Geometry check sheet. Reference: the model listing, model coordinates, mm. Face numbers are marked on the shaded views. Coordinates: 2 decimals unless noted, no trailing zeros. Loops run counter-clockwise (first coordinate to the right, second up) from the corner with the lowest first, then second, coordinate; pieces in that order, holes last. Notation, with made-up numbers: (25.5, -4) -> (79.5, -4) arc R13 cw to (79.5, 1) -> close; hole circle Ø4 at (6.5, -25.5). An arc over 180 degrees is marked (long way). Answer as a JSON object with one key per item and string values.
from build123d import *

# Parameters (mm, degrees)
SKETCH_1_W                       = 240
SKETCH_1_H                       = 160
EXTRUDE_1_DEPTH                  = 32
SKETCH_3_R                       = 13.5
CUT_EXTRUDE_2_DEPTH              = 291.213714355
PATTERN_LINEAR_5_COUNT           = 2
PATTERN_LINEAR_5_PITCH           = 80
PATTERN_LINEAR_6_COUNT           = 2
PATTERN_LINEAR_6_PITCH           = 80
PATTERN_LINEAR_7_COUNT           = 2
PATTERN_LINEAR_7_PITCH           = 80
PATTERN_LINEAR_7_COPY_1_SKETCH_R = 13.5
PATTERN_LINEAR_7_COPY_1_DEPTH    = 291.213714355
PATTERN_LINEAR_7_COPY_2_SKETCH_R = 13.5
PATTERN_LINEAR_7_COPY_2_DEPTH    = 291.213714355


with BuildPart() as part:
    # 草图1 → 凸台-拉伸1 (new body)
    with BuildSketch(Plane(origin=(0, 0, 0), x_dir=(1, 0, 0), z_dir=(0, 1, 0))):
        with Locations((120, 80)):
            Rectangle(SKETCH_1_W, SKETCH_1_H)
    extrude(amount=EXTRUDE_1_DEPTH)

    # 草图3 → 切除-拉伸2 (cut, through all)
    with BuildSketch(Plane(origin=(0, 32, 0), x_dir=(1, 0, 0), z_dir=(0, 1, 0))):
        with Locations(Location((120, 120, 0), (0, 0, 270))):
            Circle(SKETCH_3_R)
    cut_extrude_2 = extrude(amount=-CUT_EXTRUDE_2_DEPTH, mode=Mode.SUBTRACT)

    # 阵列(线性)5: 切除-拉伸2 ×2
    with Locations(*[(-i * PATTERN_LINEAR_5_PITCH, 0, 0) for i in range(1, PATTERN_LINEAR_5_COUNT)]):
        add(cut_extrude_2, mode=Mode.SUBTRACT)

    # 阵列(线性)6: 切除-拉伸2 ×2
    with Locations(*[(i * PATTERN_LINEAR_6_PITCH, 0, 0) for i in range(1, PATTERN_LINEAR_6_COUNT)]):
        add(cut_extrude_2, mode=Mode.SUBTRACT)

    # 阵列(线性)7: 切除-拉伸2 ×2
    with Locations(*[(0, 0, i * PATTERN_LINEAR_7_PITCH) for i in range(1, PATTERN_LINEAR_7_COUNT)]):
        add(cut_extrude_2, mode=Mode.SUBTRACT)

    # 阵列(线性)7 copy 1 sketch → 阵列(线性)7 copy 1 (cut, through all)
    with BuildSketch(Plane(origin=(-80, 32, 80), x_dir=(1, 0, 0), z_dir=(0, 1, 0))):
        with Locations(Location((120, 120, 0), (0, 0, 270))):
            Circle(PATTERN_LINEAR_7_COPY_1_SKETCH_R)
    extrude(amount=-PATTERN_LINEAR_7_COPY_1_DEPTH, mode=Mode.SUBTRACT)

    # 阵列(线性)7 copy 2 sketch → 阵列(线性)7 copy 2 (cut, through all)
    with BuildSketch(Plane(origin=(80, 32, 80), x_dir=(1, 0, 0), z_dir=(0, 1, 0))):
        with Locations(Location((120, 120, 0), (0, 0, 270))):
            Circle(PATTERN_LINEAR_7_COPY_2_SKETCH_R)
    extrude(amount=-PATTERN_LINEAR_7_COPY_2_DEPTH, mode=Mode.SUBTRACT)


solid = part.part
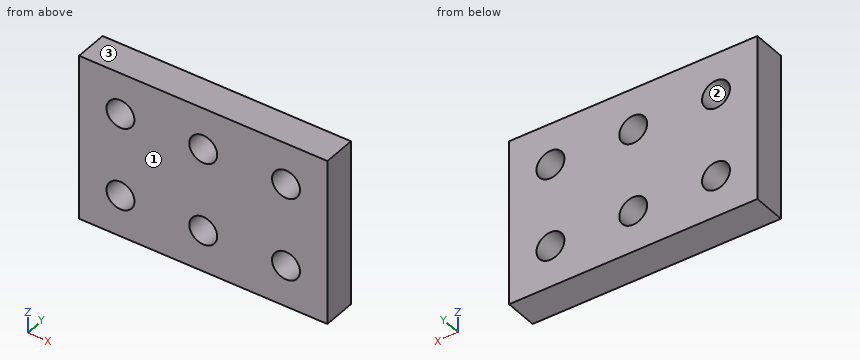
1. Section check A-A, the plane z = -120. Record the boundary of the cut face in (x, y), then the cut area to 3 significant figures.
Evaluation:
{"outline": "(0, 0) -> (26.5, 0) -> (26.5, 32) -> (0, 32) -> close; (53.5, 0) -> (106.5, 0) -> (106.5, 32) -> (53.5, 32) -> close; (133.5, 0) -> (186.5, 0) -> (186.5, 32) -> (133.5, 32) -> close; (213.5, 0) -> (240, 0) -> (240, 32) -> (213.5, 32) -> close", "area": "5,090 mm^2"}
2. Section check B-B, the plane x = 200. Record the boundary of the cut face in (y, z), then the cut area to 3 significant figures.
Evaluation:
{"outline": "(0, -160) -> (32, -160) -> (32, -133.5) -> (0, -133.5) -> close; (0, -106.5) -> (32, -106.5) -> (32, -53.5) -> (0, -53.5) -> close; (0, -26.5) -> (32, -26.5) -> (32, 0) -> (0, 0) -> close", "area": "3,390 mm^2"}
3. Mould release check, pull along Z, two halves, no side actions. Record for the marked faces 1, 2 and 3: released by +Z, released by -Z, zero draft, split by the parting line, or undercut.
Evaluation:
{"face 1": "zero draft", "face 2": "undercut", "face 3": "released by +Z"}
4. Section check C-C, the plane y = 27. Record the boundary of the cut face in (x, z), then the cut area to 3 significant figures.
Evaluation:
{"outline": "(0, -160) -> (240, -160) -> (240, 0) -> (0, 0) -> close; hole circle Ø27 at (40, -120); hole circle Ø27 at (40, -40); hole circle Ø27 at (120, -120); hole circle Ø27 at (120, -40); hole circle Ø27 at (200, -120); hole circle Ø27 at (200, -40)", "area": "35,000 mm^2"}
5. Section check D-D, the plane x = 123.5. Record the boundary of the cut face in (y, z).
Evaluation:
{"outline": "(0, -160) -> (32, -160) -> (32, -133.04) -> (0, -133.04) -> close; (0, -106.96) -> (32, -106.96) -> (32, -53.04) -> (0, -53.04) -> close; (0, -26.96) -> (32, -26.96) -> (32, 0) -> (0, 0) -> close"}
6. Thickness scan on probe 1 along X at (y, z) = (25, -40); probe 2 along X at (y, z) = (28, -115); probe 3 along Z at (x, y) = (47.5, 10.5). Record the ranges inside material, lowest first. Write a range as from..to.
Evaluation:
{"probe 1": "x = 0..26.5, 53.5..106.5, 133.5..186.5, 213.5..240", "probe 2": "x = 0..27.46, 52.54..107.46, 132.54..187.46, 212.54..240", "probe 3": "z = -160..-131.22, -108.78..-51.22, -28.78..0"}
